Verification items for the finished model (mm, model axes). Coordinates: 2 decimals unless noted, no trailing zeros. Write each loop counter-clockwise with the first axis right and the second up, starting at its lowest first coordinate (ties: lowest second). Pieces come first, ordered by that corner, then holes. Notation, with made-up numbers: (20, -30.75) - (63, -30.75) arc R16 ccw to (63, -9.75) - close; hole circle Ø1 at (-31, 51). An arc over 180 degrees is marked (long way). Use one line per item in the form item = value. Start each with the question number.
(1) Sectioned sample at C-C (z = 2.5). Record the cut outline in (x, y) (3 decimals).
(2) Sectioned sample at B-B (x = -8). Record the cut outline in (y, z) (3 decimals).
(3) Sectioned sample at A-A (y = -26). Record the cut outline in (x, z).
(4) Sectioned sample at D-D (x = 17). Record the cut outline in (y, z) (3 decimals), and give its area (3 significant figures).
(5) Material ranges on line 1 (X direction, y = 14, z = 3); line 2 (Y direction, x = -15, z = 4.25) (3 decimals); line 3 (X direction, y = 30.5, z = 4.25), recorded low to high. Write a range as [from, to].
(6) Gauge pin test, flat end, axial feed: pin 1 Ø6 at (x, y) = (-16.764, 32.004) entering from +Z. Record the tip position at first contact, or that the pin passes through.
from build123d import *

# Parameters (mm, degrees)
F0_W     = 76.2
F0_H     = 151.13
F0_R     = 2.286
F1_DEPTH = 6.35


with BuildPart() as f1:
    # F0 (on Top) → F1 (new body)
    with BuildSketch(Plane.XY):
        Rectangle(F0_W, F0_H)
        Polygon((0, 35.56), (20.32, 35.56), (20.32, 15.24), (20.32, -15.24), (20.32, -35.56), (0, -35.56), (-20.32, -35.56), (-20.32, -15.24), (-20.32, 15.24), (-20.32, 35.56), align=None, mode=Mode.SUBTRACT)
        with BuildLine():
            ThreePointArc((0, -35.56), (-14.36841, -29.60841), (-20.32, -15.24))
            Line((-20.32, -15.24), (-20.32, -35.56))
            Line((-20.32, -35.56), (0, -35.56))
        make_face()
        with Locations((-16.764, -32.004)):
            Circle(F0_R, mode=Mode.SUBTRACT)
        with BuildLine():
            Line((20.32, -35.56), (20.32, -15.24))
            ThreePointArc((20.32, -15.24), (14.36841, -29.60841), (0, -35.56))
            Line((0, -35.56), (20.32, -35.56))
        make_face()
        with Locations((16.764, -32.004)):
            Circle(F0_R, mode=Mode.SUBTRACT)
        with BuildLine():
            ThreePointArc((-20.32, 15.24), (-14.36841, 29.60841), (0, 35.56))
            Line((0, 35.56), (-20.32, 35.56))
            Line((-20.32, 35.56), (-20.32, 15.24))
        make_face()
        with Locations((-16.764, 32.004)):
            Circle(F0_R, mode=Mode.SUBTRACT)
        with BuildLine():
            Line((20.32, 15.24), (20.32, 35.56))
            Line((20.32, 35.56), (0, 35.56))
            ThreePointArc((0, 35.56), (14.36841, 29.60841), (20.32, 15.24))
        make_face()
        with Locations((16.764, 32.004)):
            Circle(F0_R, mode=Mode.SUBTRACT)
    extrude(amount=F1_DEPTH)


solid = f1.part
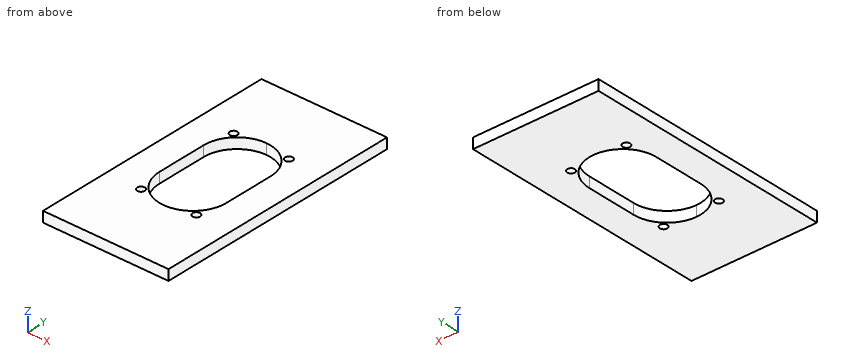
Answers below:
q1.outline = (-38.1, -75.565) - (38.1, -75.565) - (38.1, 75.565) - (-38.1, 75.565) - close; hole (-20.32, -15.24) arc R20.32 ccw to (0, -35.56) arc R20.32 ccw to (20.32, -15.24) - (20.32, 15.24) arc R20.32 ccw to (0, 35.56) arc R20.32 ccw to (-20.32, 15.24) - close; hole circle Ø4.572 at (-16.764, -32.004); hole circle Ø4.572 at (-16.764, 32.004); hole circle Ø4.572 at (16.764, -32.004); hole circle Ø4.572 at (16.764, 32.004)
q2.outline = (-75.565, 0) - (-33.919, 0) - (-33.919, 6.35) - (-75.565, 6.35) - close; (33.919, 0) - (75.565, 0) - (75.565, 6.35) - (33.919, 6.35) - close
q3.outline = (-38.1, 0) - (-17.24, 0) - (-17.24, 6.35) - (-38.1, 6.35) - close; (17.24, 0) - (38.1, 0) - (38.1, 6.35) - (17.24, 6.35) - close
q4.outline = (-75.565, 0) - (-34.278, 0) - (-34.278, 6.35) - (-75.565, 6.35) - close; (-29.73, 0) - (-26.371, 0) - (-26.371, 6.35) - (-29.73, 6.35) - close; (26.371, 0) - (29.73, 0) - (29.73, 6.35) - (26.371, 6.35) - close; (34.278, 0) - (75.565, 0) - (75.565, 6.35) - (34.278, 6.35) - close
q4.area = 567 mm2
q5.line_1 = [-38.1, -20.32], [20.32, 38.1]
q5.line_2 = [-75.565, -33.458], [-30.55, -28.948], [28.948, 30.55], [33.458, 75.565]
q5.line_3 = [-38.1, -18.49], [-15.04, -13.42], [13.42, 15.04], [18.49, 38.1]
q6.pin_1 = 6.35
